```python
from build123d import *
from OCP.BRepFilletAPI import BRepFilletAPI_MakeChamfer

# Parameters (mm, degrees)
SKETCH1_W           = 81.28
SKETCH1_H           = 55.88
SKETCH1_W_2         = 76.2
SKETCH1_H_2         = 50.8
BOSS_EXTRUDE1_DEPTH = 28.575
SKETCH2_W           = 81.28
SKETCH2_H           = 55.88
BOSS_EXTRUDE2_DEPTH = 2.54
SKETCH5_W           = 13.208
SKETCH5_H           = 12.192
CUT_EXTRUDE1_DEPTH  = 2.54
SKETCH6_R           = 12.7
CUT_EXTRUDE2_DEPTH  = 2.54
CHAMFER4_SIZE       = 1.052102448
CHAMFER4_SIZE_2     = 2.54
CUT_EXTRUDE3_DEPTH  = 2.54
CHAMFER5_SIZE       = 2.54
FILLET2_R           = 0.762
FILLET3_R           = 2.54


with BuildPart() as part:
    # Sketch1 → Boss-Extrude1 (new body)
    with BuildSketch(Plane.XY):
        with Locations((2.94888724, 5.055504451)):
            Rectangle(SKETCH1_W, SKETCH1_H)
        with Locations((2.94888724, 5.055504451)):
            Rectangle(SKETCH1_W_2, SKETCH1_H_2, mode=Mode.SUBTRACT)
    extrude(amount=BOSS_EXTRUDE1_DEPTH)

    # Sketch2 → Boss-Extrude2 (add)
    with BuildSketch(Plane.XY.offset(28.575)):
        with Locations((2.94888724, 5.055504451)):
            Rectangle(SKETCH2_W, SKETCH2_H)
    extrude(amount=BOSS_EXTRUDE2_DEPTH)

    # Sketch5 → Cut-Extrude1 (cut)
    with BuildSketch(Plane(origin=(43.58888724, 0, 0), x_dir=(0, 0, -1), z_dir=(1, 0, 0))):
        with Locations((-12.954, -11.073495549)):
            Rectangle(SKETCH5_W, SKETCH5_H)
    extrude(amount=-CUT_EXTRUDE1_DEPTH, mode=Mode.SUBTRACT)

    # Sketch6 → Cut-Extrude2 (cut)
    with BuildSketch(Plane(origin=(0, 32.995504451, 0), x_dir=(1, 0, 0), z_dir=(0, 1, 0))):
        with Locations((2.94888724, -3.175)):
            Circle(SKETCH6_R)
    extrude(amount=-CUT_EXTRUDE2_DEPTH, mode=Mode.SUBTRACT)

    # Chamfer4
    chamfer4_edges_1 = [part.edges().sort_by_distance(p)[0] for p in [
        (41.04888724, -17.169495549, 12.954),
    ]]
    chamfer4_side_1 = [part.faces().sort_by_distance(p)[0] for p in [
        (41.04888724, -17.190537598, 12.954),
    ]]
    chamfer4_edges_2 = [part.edges().sort_by_distance(p)[0] for p in [
        (41.04888724, -11.073495549, 19.558),
    ]]
    chamfer4_side_2 = [part.faces().sort_by_distance(p)[0] for p in [
        (41.04888724, -11.073495549, 19.579042049),
    ]]
    chamfer4_edges_3 = [part.edges().sort_by_distance(p)[0] for p in [
        (41.04888724, -4.977495549, 12.954),
    ]]
    chamfer4_side_3 = [part.faces().sort_by_distance(p)[0] for p in [
        (41.04888724, -4.9564535, 12.954),
    ]]
    chamfer4_edges_4 = [part.edges().sort_by_distance(p)[0] for p in [
        (41.04888724, -11.073495549, 6.35),
    ]]
    chamfer4_side_4 = [part.faces().sort_by_distance(p)[0] for p in [
        (41.04888724, -11.073495549, 6.328957951),
    ]]
    chamfer4 = BRepFilletAPI_MakeChamfer(part.part.solid().wrapped)
    for e in chamfer4_edges_1:
        chamfer4.Add(CHAMFER4_SIZE - 0.0001, CHAMFER4_SIZE_2 - 0.0001, e.wrapped, chamfer4_side_1[0].wrapped)
    for e in chamfer4_edges_2:
        chamfer4.Add(CHAMFER4_SIZE - 0.0001, CHAMFER4_SIZE_2 - 0.0001, e.wrapped, chamfer4_side_2[0].wrapped)
    for e in chamfer4_edges_3:
        chamfer4.Add(CHAMFER4_SIZE - 0.0001, CHAMFER4_SIZE_2 - 0.0001, e.wrapped, chamfer4_side_3[0].wrapped)
    for e in chamfer4_edges_4:
        chamfer4.Add(CHAMFER4_SIZE - 0.0001, CHAMFER4_SIZE_2 - 0.0001, e.wrapped, chamfer4_side_4[0].wrapped)
    add(Compound.cast(chamfer4.Shape()), mode=Mode.REPLACE)  # a hair under: the kernel refuses the full size

    # Sketch8 → Cut-Extrude3 (cut)
    with BuildSketch(Plane(origin=(0, 0, 0), x_dir=(-1, 0, 0), z_dir=(0, 0, -1))):
        Polygon((-41.04888724, 30.455504451), (-21.99888724, 30.455504451), (-21.99888724, 31.725504451), (-42.31888724, 31.725504451), (-42.31888724, -21.614495549), (36.42111276, -21.614495549), (36.42111276, 31.725504451), (16.10111276, 31.725504451), (16.10111276, 30.455504451), (35.15111276, 30.455504451), (35.15111276, -20.344495549), (-41.04888724, -20.344495549), align=None)
    extrude(amount=-CUT_EXTRUDE3_DEPTH, mode=Mode.SUBTRACT)

    # Chamfer5
    chamfer5_edges = [part.edges().sort_by_distance(p)[0] for p in [
        (2.94888724, 30.455504451, 15.875),
    ]]
    chamfer(chamfer5_edges, length=CHAMFER5_SIZE - 0.0001)  # a hair under: the kernel refuses the full size

    # Fillet2
    fillet2_edges = [part.edges().sort_by_distance(p)[0] for p in [
        (32.15888724, 31.725504451, 0),
        (42.31888724, 5.055504451, 0),
        (2.94888724, -21.614495549, 0),
        (-36.42111276, 5.055504451, 0),
        (-26.26111276, 31.725504451, 0),
    ]]
    fillet(fillet2_edges, radius=FILLET2_R)

    # Fillet3
    fillet3_edges = [part.edges().sort_by_distance(p)[0] for p in [
        (-37.69111276, 5.055504451, 31.115),
        (2.94888724, -22.884495549, 31.115),
        (43.58888724, 5.055504451, 31.115),
        (2.94888724, 32.995504451, 31.115),
    ]]
    fillet(fillet3_edges, radius=FILLET3_R)


solid = part.part
```
Verification items for the finished model (mm, model axes). A direction names the side the tool comes from. Coordinates: 2 decimals unless noted, no trailing zeros. Write each loop counter-clockwise with the first axis right and the second up, starting at its lowest first coordinate (ties: lowest second). Pieces come first, ordered by that corner, then holes. Notation, with made-up numbers: (-29.5, -23.75) - (9.5, -23.75) arc R18 cw to (9.5, -9.75) - close; hole circle Ø5 at (18, 52). An arc over 180 degrees is marked (long way). One line per question, with ' | ' between items. Start each with the question number.
1. Material ranges on line 1 along Y through (x, z) = (-26.5, 16.5); line 2 along X through (y, z) = (-4, 24); line 3 along Z through (x, y) = (32, 2) (3 decimals), recorded low to high.
2. Section check B-B (z = 22.5). Enter the section's corners in (x, y).
3. Access from +Z, -Z, +X, -X, +Y, -Y to the whole of each face (thin tool, end or side, straight path). Record for faces 1 (the flat face through (2, -20.344, 15)), 2 (the flat face through (42.337, -11.174, 5.831)), 3 (the flat face through (2, 5, 31.115)).
4. Section check D-D (y = 9.5). Enter the section's corners in (x, z) (3 decimals), plus the area to 3 significant figures.
5. Draft check along X on faces 4 (the cylindrical face through (42.865, 5.447, 30.351)), 5 (the flat face through (4, -21.614, 2)), 6 (the flat face through (42.34, -4.46, 13.06)), 7 (the cylindrical face through (3.52, 32.23, 30.39)). Enter one of: released by +X, released by -X, zero draft, split by the parting line, or undercut.
6. Gauge pin test, flat ends, axial feed: P1, Ø10, axis at x = 20, y = -16.5, coming from the -Z side; P2, Ø12, axis at x = -27, y = -12, coming from the -Z side (3 decimals); P3, Ø2, axis at x = 9, z = 2, coming from the +Y side. Record the tip position at first contact, or that the pin passes through.
7. Section check C-C (x = -30). Enter the section's corners in (y, z) (1 decimal).
Computed values:
1) line 1: -22.88 to -20.34, 30.46 to 33 | line 2: -37.69 to -35.15, 41.05 to 43.59 | line 3: 28.575 to 31.115
2) outline: (-37.69, -22.88) - (43.59, -22.88) - (43.59, 33) - (-37.69, 33) - close; hole (-35.15, -20.34) - (41.05, -20.34) - (41.05, 30.46) - (-35.15, 30.46) - close
3) face 1: -Z | face 2: none | face 3: +Z, +X, -X, +Y, -Y
4) outline: (-37.691, 0) - (-37.183, 0) arc R0.762 ccw to (-36.421, 0.762) - (-36.421, 2.54) - (-35.151, 2.54) - (-35.151, 28.575) - (41.049, 28.575) - (41.049, 2.54) - (42.319, 2.54) - (42.319, 0.762) arc R0.762 ccw to (43.081, 0) - (43.589, 0) - (43.589, 28.575) arc R2.54 ccw to (41.049, 31.115) - (-35.151, 31.115) arc R2.54 ccw to (-37.691, 28.575) - close | area: 342 mm²
5) face 4: released by +X | face 5: undercut | face 6: undercut | face 7: zero draft
6) P1: z = 2.54 | P2: z = 28.575 | P3: y = -20.34
7) outline: (-22.9, 0) - (-22.4, 0) arc R0.8 ccw to (-21.6, 0.8) - (-21.6, 2.5) - (-20.3, 2.5) - (-20.3, 28.6) - (30.5, 28.6) - (30.5, 2.5) - (31.7, 2.5) - (31.7, 0.8) arc R0.8 ccw to (32.5, 0) - (33, 0) - (33, 28.6) arc R2.5 ccw to (30.5, 31.1) - (-20.3, 31.1) arc R2.5 ccw to (-22.9, 28.6) - close
